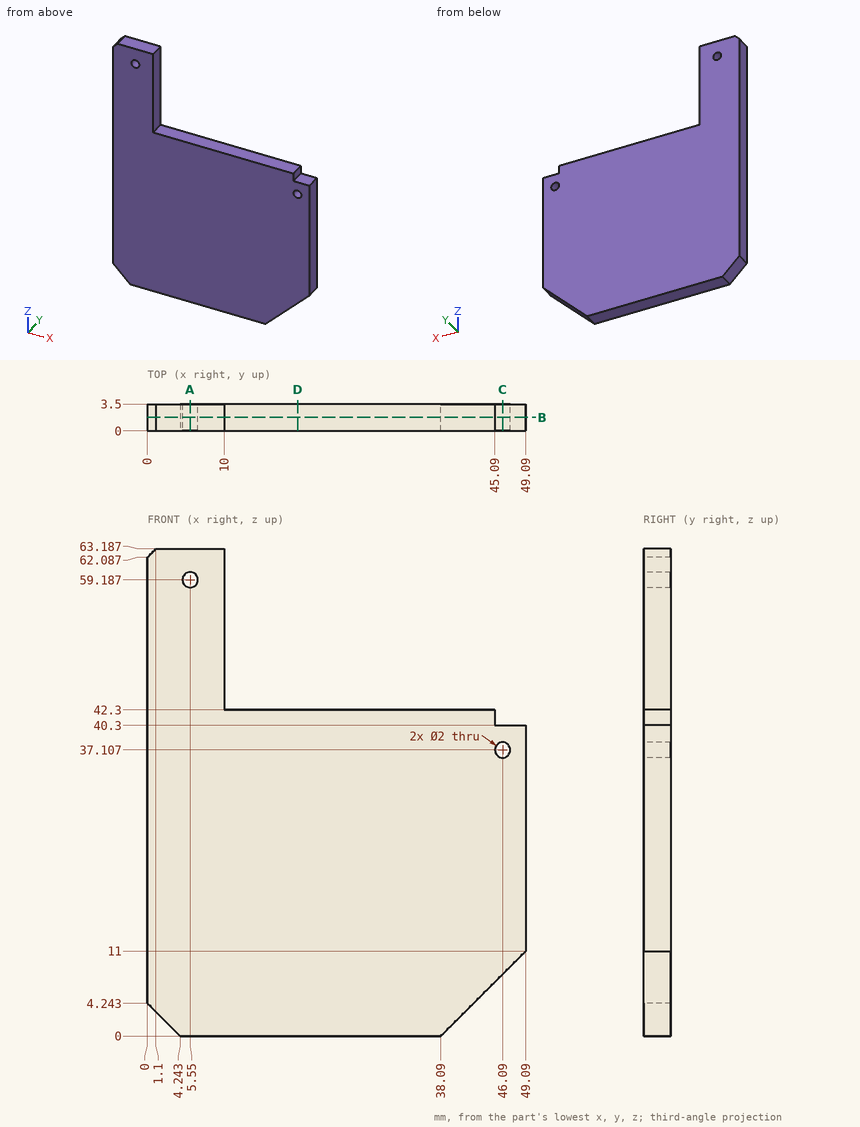
Source: three-view drawing plus pictorial views. Frame: mm from the lowest corner of the part. Round coordinates to 2 decimals unless told otherwise and drop trailing zeros. Write each loop counter-clockwise with the first axis right and the second up, starting at its lowest first coordinate (ties: lowest second). Pieces come first, ordered by that corner, then holes. Notation, with made-up numbers: (-5.75, 34.5) -> (53.25, 34.5) arc R7 cw to (53.25, 44.5) -> close; hole circle Ø9 at (-28, 3). An arc over 180 degrees is marked (long way). Return JSON: item names as keys, results as strings.
Q1. Section D-D on x = 19.5. Return the cut outline in (y, z).
From the geometry:
{"outline": "(0, 0) -> (3.5, 0) -> (3.5, 42.3) -> (0, 42.3) -> close"}
Q2. First-contact query: pin 1 Ø1.6 at (x, z) = (5.55, 59.19) entering from -Y; pin 2 Ø1.8 at (y, z) = (1.5, 49) entering from +X; pin 3 Ø1.8 at (x, y) = (23.5, 1) entering from +Z; pin 4 Ø2 at (y, z) = (2, 41.5) entering from +X. Flat tips, straight axial feed; report the tip coordinate or a pass-through.
From the geometry:
{"pin 1": "through", "pin 2": "x = 10", "pin 3": "z = 42.3", "pin 4": "x = 45.09"}
Q3. Section B-B on y = 1.75. Return the cut outline in (x, z).
From the geometry:
{"outline": "(0, 4.24) -> (4.24, 0) -> (38.09, 0) -> (49.09, 11) -> (49.09, 40.3) -> (45.09, 40.3) -> (45.09, 42.3) -> (10, 42.3) -> (10, 63.19) -> (1.1, 63.19) -> (0, 62.09) -> close; hole circle Ø2 at (5.55, 59.19); hole circle Ø2 at (46.09, 37.11)"}
Q4. Section A-A on x = 5.55. Return the cut outline in (y, z).
From the geometry:
{"outline": "(0, 0) -> (3.5, 0) -> (3.5, 58.19) -> (0, 58.19) -> close; (0, 60.19) -> (3.5, 60.19) -> (3.5, 63.19) -> (0, 63.19) -> close"}
Q5. Section C-C on x = 46.09. Return the cut outline in (y, z), and give its area (3 significant figures).
From the geometry:
{"outline": "(0, 8) -> (3.5, 8) -> (3.5, 36.11) -> (0, 36.11) -> close; (0, 38.11) -> (3.5, 38.11) -> (3.5, 40.3) -> (0, 40.3) -> close", "area": "106 mm2"}
Q6. Ray query, line 1 (Z direction, x = 5.55, y = 1.9); line 2 (X direction, y = 0.3, z = 7); line 3 (Z direction, x = 26, y = 2.05). Return the intervals inside material, ascending.
From the geometry:
{"line 1": "0 to 58.19, 60.19 to 63.19", "line 2": "0 to 45.09", "line 3": "0 to 42.3"}
